Source: CAD feature listing. Evaluate the final solid. Frame: model axes, mm. A direction names the side the tool comes from. Give positions to 0.01 mm unless a question says otherwise; leave off trailing zeros. Loops run counter-clockwise (first coordinate to the right, second up) from the corner with the lowest first, then second, coordinate; pieces in that order, holes last. Notation, with made-up numbers: (-38.5, 47) -> (-21.5, 47) arc R24 ccw to (-21.5, 70) -> close; hole circle Ø4 at (33, 71.5). An arc over 180 degrees is marked (long way). Return JSON: item names as keys, results as strings. Group by question number.
(1) Ray query, line 1 (Z direction, x = 23, y = -19); line 2 (Y direction, x = 6, z = -1.5); line 3 (X direction, y = 33, z = -1.5). Return the intervals inside material, ascending. Write a range as from..to.
(2) Pin query (flat end, axial travel): pin 1 (1 mm diameter, centred on x = 10, z = -1.5, fed in from +Y); pin 2 (1 mm diameter, centred on y = 80.5, z = 9.5, fed in from +X); pin 3 (0.6 mm diameter, centred on x = 15.5, z = -1, fed in from -Y); pin 4 (1.7 mm diameter, centred on y = 56, z = -0.5, fed in from +X). Return the tip coordinate at first contact, or that it passes through.
(3) Cut plane B-B on y = 54.5. Return loops of the section in (x, z), then the cut area to 3 significant figures.
(4) Cut plane C-C on y = 12. Return loops of the section in (x, z), then the cut area to 3 significant figures.
(5) Access query for faces 1 (the face through (0, 77.32, -1.06)), 2 (the face through (-0.07, 15.95, -1.06)), 3 (the face through (30.07, 77.25, -1.06)). Directions: +Z, -Z, +X, -X, +Y, -Y. A direction counts if a zero-diameter tool reaches every point of the face in a straight line with its end or side. Return the directions, or none.
(6) Cut plane A-A on x = 18. Return loops of the section in (y, z), then the cut area to 3 significant figures.
```python
from build123d import *

# Parameters (mm, degrees)
SKETCH_1_W          = 77
SKETCH_1_H          = 163.5
EXTRUDE_1_DEPTH     = 11
SKETCH_2_W          = 33
SKETCH_2_H          = 64.3
EXTRUDE_2_DEPTH     = 2.1
FILLET_1_R          = 5
FILLET_2_R          = 5
SKETCH_3_W          = 32
SKETCH_3_H          = 2
CUT_EXTRUDE_1_DEPTH = 2
WRAP_1_OUTLINE_R    = 1
WRAP_1_DEPTH        = 0.01


# Read off the part's stored shape, not the designer's step: 包覆1
with BuildPart() as part:
    # 草图1 → 凸台-拉伸1 (new body)
    with BuildSketch(Plane.XY):
        Rectangle(SKETCH_1_W, SKETCH_1_H)
    extrude(amount=EXTRUDE_1_DEPTH)

    # 草图2 → 凸台-拉伸2 (add)
    with BuildSketch(Plane(origin=(0, 0, 0), x_dir=(-1, 0, 0), z_dir=(0, 0, -1))):
        with Locations((-15, 46.6)):
            Rectangle(SKETCH_2_W, SKETCH_2_H)
    extrude(amount=EXTRUDE_2_DEPTH)

    # 圆角1
    fillet_1_edges = [part.edges().sort_by_distance(p)[0] for p in [
        (31.5, 78.75, -1.05),
        (31.5, 14.45, -1.05),
        (-1.5, 14.45, -1.05),
        (-1.5, 78.75, -1.05),
    ]]
    fillet(fillet_1_edges, radius=FILLET_1_R)

    # 圆角2
    fillet_2_edges = [part.edges().sort_by_distance(p)[0] for p in [
        (38.5, -81.75, 5.5),
        (-38.5, -81.75, 5.5),
        (-38.5, 81.75, 5.5),
        (38.5, 81.75, 5.5),
    ]]
    fillet(fillet_2_edges, radius=FILLET_2_R)

    # 草图3 → 切除-拉伸1 (cut)
    with BuildSketch(Plane.XY.offset(11)):
        with Locations((0, 80.25)):
            Rectangle(SKETCH_3_W, SKETCH_3_H)
    extrude(amount=-CUT_EXTRUDE_1_DEPTH, mode=Mode.SUBTRACT)

    # 包覆1 outline → 包覆1 (add)
    with BuildSketch(Plane(origin=(0, 0, 0), x_dir=(-1, 0, 0), z_dir=(0, 0, -1))):
        Circle(WRAP_1_OUTLINE_R)
    extrude(amount=WRAP_1_DEPTH)


solid = part.part
```
Answers:
{
 "1": {"line 1": "0..11", "line 2": "14.45..78.75", "line 3": "-1.5..31.5"},
 "2": {"pin 1": "y = 78.75", "pin 2": "x = 37.3", "pin 3": "y = 14.45", "pin 4": "x = 38.5"},
 "3": {"outline": "(-38.5, 0) -> (-1.5, 0) -> (-1.5, -2.1) -> (31.5, -2.1) -> (31.5, 0) -> (38.5, 0) -> (38.5, 11) -> (-38.5, 11) -> close", "area": "916 mm²"},
 "4": {"outline": "(-38.5, 0) -> (38.5, 0) -> (38.5, 11) -> (-38.5, 11) -> close", "area": "847 mm²"},
 "5": {"face 1": "-Z, -X, +Y", "face 2": "-Z, -X, -Y", "face 3": "-Z, +X, +Y"},
 "6": {"outline": "(-81.75, 0) -> (14.45, 0) -> (14.45, -2.1) -> (78.75, -2.1) -> (78.75, 0) -> (81.75, 0) -> (81.75, 11) -> (-81.75, 11) -> close", "area": "1,930 mm²"}
}
